from build123d import *

# Parameters (mm, degrees)
F0_R      = 18.5
F0_R_2    = 16.5
F1_DEPTH  = 26.5
F2_DEPTH  = 23
F3_R      = 6
F3_R_2    = 3
F4_DEPTH  = 6
F5_DEPTH  = 21
F7_DEPTH  = 12
F3_R_3    = 1.5
F8_DEPTH  = 10
F10_COUNT = 6
F11_R     = 3.75
F11_R_2   = 1.5
F12_DEPTH = 3
F13_DEPTH = 7


with BuildPart() as f1:
    # F0 (on Front) → F1 (new body)
    with BuildSketch(Plane.XZ):
        Circle(F0_R)
        Circle(F0_R_2, mode=Mode.SUBTRACT)
        Circle(F0_R_2)
    extrude(amount=F1_DEPTH)

    # F0 (on Front) → F2 (join)
    with BuildSketch(Plane.XZ):
        Circle(F0_R_2)
    extrude(amount=-F2_DEPTH)

    # F3 (on face) → F4 (join)
    with BuildSketch(Plane.XZ.offset(26.5)):
        with Locations((0, 7.3)):
            Circle(F3_R)
        with Locations((0, 7.3)):
            Circle(F3_R_2, mode=Mode.SUBTRACT)
    extrude(amount=F4_DEPTH)

    # F5 (add): a face of the model
    f5_faces = [f1.faces().sort_by_distance(p)[0] for p in [
        (0, -26.5, 7.3),
    ]]
    extrude(f5_faces, amount=F5_DEPTH)

    # F6 (on face) → F7 (cut)
    with BuildSketch(Plane.XZ.offset(47.5)):
        with BuildLine():
            Line((1.6583123952, 4.8), (-1.6583123952, 4.8))
            ThreePointArc((-1.6583123952, 4.8), (0, 4.3), (1.6583123952, 4.8))
        make_face()
    extrude(amount=-F7_DEPTH, mode=Mode.SUBTRACT)

    # F10: F8 ×6 about axis
    f10_axis = Axis((0, -5.8839749545, 0), (0, 1, 0))


with BuildPart() as f8:
    # F3 (on face) → F8 (new body)
    with BuildSketch(Plane.XZ.offset(26.5)):
        with Locations((-15.5, 0)):
            Circle(F3_R_3)
    extrude(amount=-F8_DEPTH)


with BuildPart() as f1_1:
    add(f1.part)
    for i in range(1, F10_COUNT):
        add(f8.part.rotate(f10_axis, i * 360 / F10_COUNT), mode=Mode.SUBTRACT)

    # F10#seed: cut F8
    add(f8.part, mode=Mode.SUBTRACT)

    # F11 (on face) → F12 (join)
    with BuildSketch(Plane(origin=(0, 23, 0), x_dir=(-1, 0, 0), z_dir=(0, 1, 0))):
        Circle(F11_R)
        with Locations((-12.5, 0)):
            Circle(F11_R_2)
        with Locations((12.5, 0)):
            Circle(F11_R_2)
    extrude(amount=F12_DEPTH)

    # F11 (on face) → F13 (join)
    with BuildSketch(Plane(origin=(0, 23, 0), x_dir=(-1, 0, 0), z_dir=(0, 1, 0))):
        with Locations((-12.5, 0)):
            Circle(F11_R_2)
        with Locations((12.5, 0)):
            Circle(F11_R_2)
    extrude(amount=F13_DEPTH)


solid = f1_1.part
Verification items for the finished model (mm, model axes). A direction names the side the tool comes from. Give positions to 0.01 mm unless a question says otherwise; leave off trailing zeros. Order: outer loops, then holes, each group sorted by start corner. A loop starts at its lowest first (then second) coordinate and runs counter-clockwise, first axis right, second up. Notation, with made-up numbers: M -30,-35.75 L -6,-35.75 A26 ccw -6,-9.75 Z; hole C -4,45 d8. An arc over 180 degrees is marked long. Use one line per item in the form item = value. Start each with the question number.
Q1. Section check B-B (y = -21). Enter the section's corners in (x, z), then the cut area to 3 significant figures.
Q2. Section check D-D (y = -36.5). Enter the section's corners in (x, z).
Q3. Section check C-C (z = 7.3). Enter the section's corners in (x, y), then the cut area to 3 significant figures.
Q4. Section check A-A (x = 0). Enter the section's corners in (y, z).
Q5. Mould release check, pull along X, two halves, no side actions. Record for faces 4 (the flat face through (0, 26, 0)), 5 (the flat face through (0, -47.5, 8)), 6 (the cylindrical face through (15.24, 11.34, -6.32)): +X half, -X half, draft (parallel to the pull), parting line (faces both ways), or undercut.
Q6. Access from +Z, -Z, +X, -X, +Y, -Y to the whole of each face (thin tool, end or side, straight path). Record for faces 1 (the cylindrical face through (-4.01, -13.06, -18.06)), 2 (the flat face through (-17, 0, 0)), 3 (the flat face through (-3, -32.5, 6)).
Q7. Go/stop test with flat-tipped pins: pin 1 Ø1.8 at (x, z) = (-7.75, 13.42) entering from -Y; pin 2 Ø5 at (x, z) = (-15.5, 0) entering from -Y; pin 3 Ø1 at (y, z) = (-30.5, 7.5) entering from +X; pin 4 Ø18.5 at (x, z) = (-7.5, 8.5) entering from +Y. Record where each tip stops, or that it passes through.
Q8. Scan lines: line 1 along Z through (x, y) = (7.75, -18.5); line 2 along Y through (x, z) = (10.5, -3.5); line 3 along Y through (x, z) = (-10.5, -14). Record each from-to range of solid material in increasing order. Write a range as [from, to].
Evaluation:
q1.outline = C 0,0 d37; hole C -15.5,0 d3; hole C -7.75,-13.42 d3; hole C -7.75,13.42 d3; hole C 7.75,-13.42 d3; hole C 7.75,13.42 d3; hole C 15.5,0 d3
q1.area = 1,030 mm2
q2.outline = M -1.66,4.8 L 1.66,4.8 A3 ccw long Z
q3.outline = M -17,-26.5 L -6,-26.5 L -6,-32.5 L -3,-32.5 L -3,-47.5 L 3,-47.5 L 3,-32.5 L 6,-32.5 L 6,-26.5 L 17,-26.5 L 17,0 L 14.8,0 L 14.8,23 L -14.8,23 L -14.8,0 L -17,0 Z
q3.area = 1,740 mm2
q4.outline = M -47.5,4.8 L -35.5,4.8 L -35.5,4.3 L -32.5,4.3 L -32.5,1.3 L -26.5,1.3 L -26.5,-18.5 L 0,-18.5 L 0,-16.5 L 23,-16.5 L 23,-3.75 L 26,-3.75 L 26,3.75 L 23,3.75 L 23,16.5 L 0,16.5 L 0,18.5 L -26.5,18.5 L -26.5,13.3 L -32.5,13.3 L -32.5,10.3 L -47.5,10.3 Z
q5.face_4 = undercut
q5.face_5 = draft
q5.face_6 = parting line
q6.face_1 = +Y, -Y
q6.face_2 = +Y
q6.face_3 = -Y
q7.pin_1 = -16.5
q7.pin_2 = -26.5
q7.pin_3 = 6
q7.pin_4 = 30
q8.line_1 = [-16.8, -14.92], [-11.92, 11.92], [14.92, 16.8]
q8.line_2 = [-26.5, 23]
q8.line_3 = [-26.5, 0]
